Geometry check sheet. Reference: the model listing, model coordinates, mm. A direction names the side the tool comes from. Round coordinates to 2 decimals unless told otherwise and drop trailing zeros. Write each loop counter-clockwise with the first axis right and the second up, starting at its lowest first coordinate (ties: lowest second). Pieces come first, ordered by that corner, then holes. Notation, with made-up numbers: M -12.5,-25 L 0.5,-25 A19 ccw 0.5,-15 Z; hole C 33,42 d1. An arc over 180 degrees is marked long. Use a Markdown table: item, result.
```python
from build123d import *

# Parameters (mm, degrees)
RESSALTO_EXTRUS_O1_DEPTH = 5
CORTE_EXTRUS_O1_DEPTH    = 5
ESBO_O3_W                = 5
ESBO_O3_H                = 25
CORTE_EXTRUS_O3_DEPTH    = 5
CORTE_EXTRUS_O4_DEPTH    = 10
CORTE_EXTRUS_O5_DEPTH    = 5
ESBO_O6_R                = 1.5
CORTE_EXTRUS_O6_DEPTH    = 20
CORTE_EXTRUS_O7_DEPTH    = 10


with BuildPart() as part:
    # Esboço1 → Ressalto-extrusão1 (new body)
    with BuildSketch(Plane(origin=(0, 0, 0), x_dir=(1, 0, 0), z_dir=(0, 1, 0))):
        with BuildLine():
            Line((-56.5, -61.5), (56.5, -61.5))
            ThreePointArc((56.5, -61.5), (60.035533906, -60.035533906), (61.5, -56.5))
            Line((61.5, -56.5), (61.5, 56.5))
            ThreePointArc((61.5, 56.5), (60.035533906, 60.035533906), (56.5, 61.5))
            Line((56.5, 61.5), (-56.5, 61.5))
            ThreePointArc((-56.5, 61.5), (-60.035533906, 60.035533906), (-61.5, 56.5))
            Line((-61.5, 56.5), (-61.5, -56.5))
            ThreePointArc((-61.5, -56.5), (-60.035533906, -60.035533906), (-56.5, -61.5))
        make_face()
    extrude(amount=RESSALTO_EXTRUS_O1_DEPTH)

    # Esboço2 → Corte-extrusão1 (cut)
    with BuildSketch(Plane(origin=(0, 5, 0), x_dir=(1, 0, 0), z_dir=(0, 1, 0))):
        with BuildLine():
            Line((-4.765646957, 54.5), (-9.733117681, 54.5))
            ThreePointArc((-9.733117681, 54.5), (-10.98249215, 53.98249215), (-11.5, 52.733117681))
            Line((-11.5, 52.733117681), (-11.5, 40.733117681))
            ThreePointArc((-11.5, 40.733117681), (-10.98249215, 39.483743212), (-9.733117681, 38.966235362))
            Line((-9.733117681, 38.966235362), (-4.765646957, 38.966235362))
            ThreePointArc((-4.765646957, 38.966235362), (-3.516272487, 39.483743212), (-2.998764638, 40.733117681))
            Line((-2.998764638, 40.733117681), (-2.998764638, 52.733117681))
            ThreePointArc((-2.998764638, 52.733117681), (-3.516272487, 53.98249215), (-4.765646957, 54.5))
        make_face()
        with BuildLine():
            Line((4.768117681, 38.966235362), (9.733117681, 38.966235362))
            ThreePointArc((9.733117681, 38.966235362), (10.98249215, 39.483743212), (11.5, 40.733117681))
            Line((11.5, 40.733117681), (11.5, 52.733117681))
            ThreePointArc((11.5, 52.733117681), (10.98249215, 53.98249215), (9.733117681, 54.5))
            Line((9.733117681, 54.5), (4.768117681, 54.5))
            ThreePointArc((4.768117681, 54.5), (3.518743212, 53.98249215), (3.001235362, 52.733117681))
            Line((3.001235362, 52.733117681), (3.001235362, 40.733117681))
            ThreePointArc((3.001235362, 40.733117681), (3.518743212, 39.483743212), (4.768117681, 38.966235362))
        make_face()
    extrude(amount=-CORTE_EXTRUS_O1_DEPTH, mode=Mode.SUBTRACT)

    # Esboço3 → Corte-extrusão3 (cut)
    with BuildSketch(Plane(origin=(0, 5, 0), x_dir=(1, 0, 0), z_dir=(0, 1, 0))):
        with Locations((-59, -34)):
            Rectangle(ESBO_O3_W, ESBO_O3_H)
        with Locations((59, -34)):
            Rectangle(ESBO_O3_W, ESBO_O3_H)
    extrude(amount=-CORTE_EXTRUS_O3_DEPTH, mode=Mode.SUBTRACT)

    # Esboço4 → Corte-extrusão4 (cut)
    with BuildSketch(Plane(origin=(0, 5, 0), x_dir=(1, 0, 0), z_dir=(0, 1, 0))):
        Polygon((56.5, -41.5), (53, -41.5), (53, -43.3), (51.5, -43.3), (51.5, -41.5), (49.5, -41.5), (49.5, -39.5), (51.5, -39.5), (51.5, -37.7), (53, -37.7), (53, -39.5), (56.5, -39.5), align=None)
        Polygon((56.5, -26.5), (53, -26.5), (53, -24.7), (51.5, -24.7), (51.5, -26.5), (49.5, -26.5), (49.5, -28.5), (51.5, -28.5), (51.5, -30.3), (53, -30.3), (53, -28.5), (56.5, -28.5), align=None)
    corte_extrus_o4 = extrude(amount=-CORTE_EXTRUS_O4_DEPTH, mode=Mode.SUBTRACT)

    # Espelhar1: Corte-extrusão4 across plane
    add(corte_extrus_o4.mirror(Plane(origin=(0, 0, 0), x_dir=(0, 0, 1), z_dir=(1, 0, 0))), mode=Mode.SUBTRACT)

    # Esboço5 → Corte-extrusão5 (cut)
    with BuildSketch(Plane(origin=(0, 5, 0), x_dir=(1, 0, 0), z_dir=(0, 1, 0))):
        with BuildLine():
            Line((43, -42.5), (-43, -42.5))
            ThreePointArc((-43, -42.5), (-44.414213562, -41.914213562), (-45, -40.5))
            Line((-45, -40.5), (-45, -28.5))
            ThreePointArc((-45, -28.5), (-44.414213562, -27.085786438), (-43, -26.5))
            Line((-43, -26.5), (43, -26.5))
            ThreePointArc((43, -26.5), (44.414213562, -27.085786438), (45, -28.5))
            Line((45, -28.5), (45, -40.5))
            ThreePointArc((45, -40.5), (44.414213562, -41.914213562), (43, -42.5))
        make_face()
    extrude(amount=-CORTE_EXTRUS_O5_DEPTH, mode=Mode.SUBTRACT)

    # Esboço6 → Corte-extrusão6 (cut)
    with BuildSketch(Plane(origin=(0, 5, 0), x_dir=(1, 0, 0), z_dir=(0, 1, 0))):
        with Locations(Location((-51.5, 46.5, 0), (0, 0, 270))):
            Circle(ESBO_O6_R)
        with Locations(Location((51.5, 46.5, 0), (0, 0, 270))):
            Circle(ESBO_O6_R)
        with Locations(Location((31.75, -47.5, 0), (0, 0, 270))):
            Circle(ESBO_O6_R)
        with Locations(Location((-31.75, -47.5, 0), (0, 0, 270))):
            Circle(ESBO_O6_R)
    extrude(amount=-CORTE_EXTRUS_O6_DEPTH, mode=Mode.SUBTRACT)

    # Esboço7 → Corte-extrusão7 (cut)
    with BuildSketch(Plane.XZ):
        with BuildLine():
            Line((7.5, 61.5), (-7.5, 61.5))
            Line((-7.5, 61.5), (-7.5, 56.5))
            ThreePointArc((-7.5, 56.5), (-6.621320344, 54.378679656), (-4.5, 53.5))
            Line((-4.5, 53.5), (4.5, 53.5))
            ThreePointArc((4.5, 53.5), (6.621320344, 54.378679656), (7.5, 56.5))
            Line((7.5, 56.5), (7.5, 61.5))
        make_face()
    extrude(amount=-CORTE_EXTRUS_O7_DEPTH, mode=Mode.SUBTRACT)


solid = part.part
```
Item 1: Cross-section at B-B, the plane x = 31.75. Record the cut outline in (y, z).
Outcome:
| item | result |
|---|---|
| outline | M 0,-61.5 L 5,-61.5 L 5,26.5 L 0,26.5 Z; M 0,42.5 L 5,42.5 L 5,46 L 0,46 Z; M 0,49 L 5,49 L 5,61.5 L 0,61.5 Z |
Item 2: Material ranges on line 1 along X through (y, z) = (4.5, -49.5); line 2 along X through (y, z) = (0.5, 30); line 3 along X through (y, z) = (1.9, -46.5), recorded low to high. Write a range as from..to.
Outcome:
| item | result |
|---|---|
| line 1 | x = -61.5..-11.5, -3..3, 11.5..61.5 |
| line 2 | x = -56.5..-53, -51.5..-45, 45..51.5, 53..56.5 |
| line 3 | x = -61.5..-53, -50..-11.5, -3..3, 11.5..50, 53..61.5 |
Item 3: Mould release check, pull along X, two halves, no side actions. Record for faces 1 (the face through (55, 3, 39.5)), 2 (the face through (7, 3, -54.5)), 3 (the face through (56.5, 3, 34)): +X half, -X half, draft (parallel to the pull), parting line (faces both ways), or undercut.
Outcome:
| item | result |
|---|---|
| face 1 | draft |
| face 2 | undercut |
| face 3 | +X half |
Item 4: Go/stop test with flat-tipped pins: pin 1 (2 mm diameter, centred on y = 3.5, z = 42, fed in from -X); pin 2 (1.5 mm diameter, centred on x = 60, y = 2.5, fed in from +Z); pin 3 (1.5 mm diameter, centred on y = 2.5, z = 36.5, fed in from +X); pin 4 (12 mm diameter, centred on x = -27, z = 3, fed in from -Y). Record where each tip stops, or that it passes through.
Outcome:
| item | result |
|---|---|
| pin 1 | stops at x = -56.5 |
| pin 2 | stops at z = 60.68 |
| pin 3 | stops at x = 56.5 |
| pin 4 | stops at y = 0 |
Item 5: Access from +Z, -Z, +X, -X, +Y, -Y to the whole of each face (thin tool, end or side, straight path). Record for faces 4 (the face through (-1, 3, 26.5)), 5 (the face through (-55, 3, 39.5)), 6 (the face through (61.5, 2, 52)).
Outcome:
| item | result |
|---|---|
| face 4 | +Y, -Y |
| face 5 | -X, +Y, -Y |
| face 6 | +Z, -Z, +X, +Y, -Y |
Item 6: Cross-section at C-C, the plane y = 2.75. Count the separate pieces of the cut face and the enclosed holes in it, and give its area (3 significant figures).
Outcome:
| item | result |
|---|---|
| separate pieces | 1 |
| enclosed holes | 7 |
| area | 12,900 mm2 |
Item 7: Cross-section at A-A, the plane z = -46.5. Record the cut outline in (x, y), and give its area (3 significant figures).
Outcome:
| item | result |
|---|---|
| outline | M -61.5,0 L -53,0 L -53,5 L -61.5,5 Z; M -50,0 L -11.5,0 L -11.5,5 L -50,5 Z; M -3,0 L 3,0 L 3,5 L -3,5 Z; M 11.5,0 L 50,0 L 50,5 L 11.5,5 Z; M 53,0 L 61.5,0 L 61.5,5 L 53,5 Z |
| area | 500 mm2 |
